Could you check a few things on this model? Use its own coordinates, in mm. A direction names the side the tool comes from. Give positions to 0.01 mm unless a question says otherwise; leave off trailing zeros. Loops run counter-clockwise (first coordinate to the right, second up) from the corner with the lowest first, then second, coordinate; pieces in that order, holes last. Notation, with made-up numbers: (77.5, 64.25) - (97.5, 64.25) arc R22 cw to (97.5, 73.25) - close; hole circle Ø1 at (88, 32.5). An arc over 180 degrees is marked (long way). One line per item, written item: value. Start each with the question number.
Q1. For faces 5 (the face through (0, 8.5, 0)), 6 (the face through (-10, 1, 0)), 7 (the face through (1.636, 4.801, 5.195)), which set-ups out of +Z, -Z, +X, -X, +Y, -Y let a thin tool reach every point of the face, with its end or its side?
Q2. I want a section at D-D (y = 4.75). Please give me the cut outline in (x, z), then the cut area to 3 significant figures.
Q3. If we mould it in two halves opening along Z, with no side actions, what happens to faces 1 (the face through (2.6, 4.19, 1.39)), 2 (the face through (0.06, 0.74, -6.05)), 3 (the face through (5.61, 0.76, 0.15)), 4 (the face through (-0.06, 0.74, 6.05))? For each: released by +Z, released by -Z, zero draft, split by the parting line, or undercut.
Q4. I want a section at C-C (x = 7.25). Please give me the cut outline in (y, z).
Q5. I'm going to push flat-ended pins straight in: P1, Ø1.5, axis at y = 2.5, z = -1, coming from the -X side; P2, Ø1.4, axis at x = -6.75, z = 0, coming from the +Y side. Where does each tip first touch, or does it pass through?
Q6. I want a section at A-A (z = 0). Count the separate pieces of the cut face and the enclosed holes in it, then the cut area to 3 significant figures.
Q7. If I drill on line 1 (X direction, y = 0.7, z = 0); line 2 (X direction, y = 3, z = 0); line 3 (Z direction, x = 6.75, y = 0.35), over which ranges is the centre line in solid material (lowest first)? Write a range as from..to.
```python
from build123d import *

# Parameters (mm, degrees)
BOSS_EXTRUDE1_OUTLINE_R = 2.946896199
BOSS_EXTRUDE1_DEPTH     = 1.5
SKETCH2_R               = 1.15
CUT_EXTRUDE1_DEPTH      = 12.783569218
SKETCH3_R               = 5.446896199
SKETCH3_R_2             = 2.946896199
BOSS_EXTRUDE2_DEPTH     = 7
SKETCH4_R               = 4.25
BOSS_EXTRUDE3_DEPTH     = 3
FILLET1_R               = 4
FILLET2_R               = 0.5
FILLET3_R               = 0.2


# Read off the part's stored shape, not the designer's step: Boss-Extrude1
with BuildPart() as part:
    # Boss-Extrude1 outline → Boss-Extrude1 (new body)
    with BuildSketch(Plane(origin=(0, 0, 0), x_dir=(1, 0, 0), z_dir=(0, 1, 0))):
        with BuildLine():
            ThreePointArc((-6.75, 3.25), (-10, 0), (-6.75, -3.25))
            add(Edge.make_bspline(
                [(-6.75, -3.25), (-5.557172284, -3.046535522), (-4.778196117, -3.855368441), (-3.992313535, -4.545759853)],
                knots=[0, 0, 0, 0, 1, 1, 1, 1], degree=3))
            ThreePointArc((-3.992313535, -4.545759853), (0, -6.05), (3.992313535, -4.545759853))
            add(Edge.make_bspline(
                [(6.75, -3.25), (5.557172284, -3.046535522), (4.778196117, -3.855368441), (3.992313535, -4.545759853)],
                knots=[0, 0, 0, 0, 1, 1, 1, 1], degree=3))
            ThreePointArc((6.75, -3.25), (10, 0), (6.75, 3.25))
            add(Edge.make_bspline(
                [(6.75, 3.25), (5.557172284, 3.046535522), (4.778196117, 3.855368441), (3.992313535, 4.545759853)],
                knots=[0, 0, 0, 0, 1, 1, 1, 1], degree=3))
            ThreePointArc((3.992313535, 4.545759853), (0, 6.05), (-3.992313535, 4.545759853))
            add(Edge.make_bspline(
                [(-6.75, 3.25), (-5.557172284, 3.046535522), (-4.778196117, 3.855368441), (-3.992313535, 4.545759853)],
                knots=[0, 0, 0, 0, 1, 1, 1, 1], degree=3))
        make_face()
        Circle(BOSS_EXTRUDE1_OUTLINE_R, mode=Mode.SUBTRACT)
    extrude(amount=BOSS_EXTRUDE1_DEPTH)

    # Sketch2 → Cut-Extrude1 (cut, through all)
    with BuildSketch(Plane(origin=(0, 1.5, 0), x_dir=(1, 0, 0), z_dir=(0, 1, 0))):
        with Locations(Location((-6.75, 0, 0), (0, 0, 270))):
            Circle(SKETCH2_R)
        with Locations(Location((6.75, 0, 0), (0, 0, 90))):
            Circle(SKETCH2_R)
    extrude(amount=-CUT_EXTRUDE1_DEPTH, mode=Mode.SUBTRACT)

    # Sketch3 → Boss-Extrude2 (add)
    with BuildSketch(Plane(origin=(0, 1.5, 0), x_dir=(1, 0, 0), z_dir=(0, 1, 0))):
        with Locations(Location((0, 0, 0), (0, 0, 270))):
            Circle(SKETCH3_R)
        with Locations(Location((0, 0, 0), (0, 0, 270))):
            Circle(SKETCH3_R_2, mode=Mode.SUBTRACT)
    extrude(amount=BOSS_EXTRUDE2_DEPTH)

    # Sketch4 → Boss-Extrude3 (add)
    with BuildSketch(Plane(origin=(0, 8.5, 0), x_dir=(1, 0, 0), z_dir=(0, 1, 0))):
        with Locations(Location((0, 0, 0), (0, 0, 270))):
            Circle(SKETCH4_R)
    extrude(amount=BOSS_EXTRUDE3_DEPTH)

    # Fillet1
    # the kernel refuses this fillet: 4 mm, written as the material it takes off along each edge
    with BuildSketch(Plane(origin=(0, 11.5, 0), x_dir=(0, 0, 1), z_dir=(-1, 0, 0))) as fillet1_piece_1:
        with BuildLine():
            CenterArc((0.377016654, -4), FILLET1_R, 14.477512186, 75.522487814)
            Line((0.377016654, 0), (0.377016654, 0.08))
            Line((0.377016654, 0.08), (4.25, 0.08))
            Line((4.25, 0.08), (4.33, 0))
            ThreePointArc((4.33, 0), (4.33, -1.5), (4.327459667, -2.98))
            Line((4.327459667, -2.98), (4.25, -3))
        make_face()
    revolve(axis=Axis((0, 11.5, 0), (0, 1, 0)), mode=Mode.SUBTRACT)

    # Fillet2
    fillet2_edges = [part.edges().sort_by_distance(p)[0] for p in [
        (0, 8.5, -5.446896199),
    ]]
    fillet(fillet2_edges, radius=FILLET2_R)

    # Fillet3
    fillet3_edges = [part.edges().sort_by_distance(p)[0] for p in [
        (0, 1.5, -5.446896199),
    ]]
    fillet(fillet3_edges, radius=FILLET3_R)


solid = part.part
```
Worked answers:
1. face 5: -Y
1. face 6: -X, +Y, -Y
1. face 7: +Y
2. outline: circle Ø10.89 at (0, 0); hole circle Ø5.89 at (0, 0)
2. area: 65.9 mm²
3. face 1: undercut
3. face 2: released by -Z
3. face 3: undercut
3. face 4: released by +Z
4. outline: (0, -3.21) - (1.5, -3.21) - (1.5, -1.04) - (0, -1.04) - close; (0, 1.04) - (1.5, 1.04) - (1.5, 3.21) - (0, 3.21) - close
5. P1: stops at x = -5.44
5. P2: passes through
6. separate pieces: 3
6. enclosed holes: 0
6. area: 68.6 mm²
7. line 1: x = -10..-7.9, -5.6..-2.95, 2.95..5.6, 7.9..10
7. line 2: x = -5.45..-2.95, 2.95..5.45
7. line 3: z = -3.25..-1.15, 1.15..3.25
